The model under review builds one solid part; all positions refer to its coordinate system, in mm. Face numbers are marked on the shaded views. A direction names the side the tool comes from. Coordinates: 2 decimals unless noted, no trailing zeros. Write each loop counter-clockwise with the first axis right and the second up, starting at its lowest first coordinate (ties: lowest second). Pieces come first, ordered by that corner, then holes. Notation, with made-up numbers: (21, 86.25) - (50, 86.25) arc R20 cw to (50, 111.25) - close; hole circle Ø6 at (-13, 7). An arc over 180 degrees is marked (long way). Return JSON: item names as keys, results as strings. Group by question number.
(1) We need section A-A on z = -15. State the section outline as (x, y) points, then the cut area to 3 significant figures.
(2) We need section C-C on y = 3. State the section outline as (x, z) points, then the cut area to 3 significant figures.
(3) To check wall thickness, follow L1, parallel to X at y = 29, z = -6; L2, parallel to Y at x = 3, z = -28. State the ranges of each line that lie inside material, in increasing order. Write a range as from..to.
(4) We need section B-B on x = 10. State the section outline as (y, z) points, then the cut area to 3 significant figures.
(5) Tool access review of the marked faces 1 and 2: name each direction out of +Z, -Z, +X, -X, +Y, -Y from which nothing blocks a thin tool from reaching the whole face with its end or side.
(6) For pin 1 Ø10 at (y, z) = (23, -22.5) entering from +X; pin 2 Ø3 at (x, y) = (7, 35) entering from -Z, all flat-tipped, find the tip position at first contact; note any pin that passes through.
(7) We need section D-D on z = -7. State the section outline as (x, y) points, then the cut area to 3 significant figures.
```python
from build123d import *

# Parameters (mm, degrees)
F1_DEPTH = 30
F3_DEPTH = 15.3
F5_DEPTH = 25


with BuildPart() as f1:
    # F0 (on Top) → F1 (new body)
    with BuildSketch(Plane.XY):
        Polygon((4.9999998882, 40), (0, 40), (0, 0), (40, 0), (40, 4.9999998882), (4.9999998882, 4.9999998882), align=None)
    extrude(amount=-F1_DEPTH)

    # F2 (on face) → F3 (cut)
    with BuildSketch(Plane.YZ.offset(4.9999998882)):
        with BuildLine():
            Line((40, -3.8196602917), (40, 0))
            Line((40, 0), (29.9999997997, 0))
            ThreePointArc((29.9999997997, 0), (35.3523312718, -0.9874146635), (40, -3.8196602917))
        make_face()
        with BuildLine():
            Line((40, -30), (40, -26.1803397083))
            ThreePointArc((40, -26.1803397083), (35.3523313132, -29.0125853207), (29.9999998882, -30))
            Line((29.9999998882, -30), (40, -30))
        make_face()
    extrude(amount=-F3_DEPTH, mode=Mode.SUBTRACT)

    # F4 (on face) → F5 (cut)
    with BuildSketch(Plane(origin=(0, 4.9999998882, 0), x_dir=(-1, 0, 0), z_dir=(0, 1, 0))):
        with BuildLine():
            Line((-24.5546065271, 0), (-40, 0))
            Line((-40, 0), (-40, -30))
            Line((-40, -30), (-24.5546074611, -30))
            ThreePointArc((-24.5546074611, -30), (-39.5546074611, -14.999999533), (-24.5546065271, 0))
        make_face()
    extrude(amount=-F5_DEPTH, mode=Mode.SUBTRACT)


solid = f1.part
```
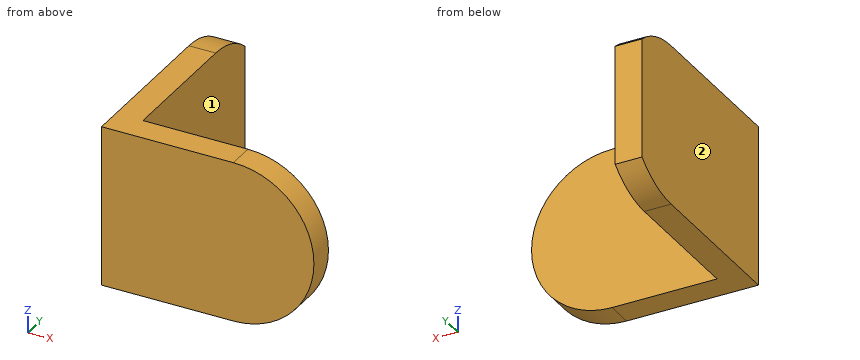
Ans:
{
 "1": {"outline": "(0, 0) - (39.55, 0) - (39.55, 5) - (5, 5) - (5, 40) - (0, 40) - close", "area": "373 mm²"},
 "2": {"outline": "(0, -30) - (24.55, -30) arc R15 ccw to (24.55, 0) - (0, 0) - close", "area": "1,090 mm²"},
 "3": {"L1": "0..5", "L2": "0..37.48"},
 "4": {"outline": "(0, -30) - (5, -30) - (5, 0) - (0, 0) - close", "area": "150 mm²"},
 "5": {"face 1": "+Z, -Z, +X, +Y", "face 2": "+Z, -Z, -X, +Y, -Y"},
 "6": {"pin 1": "x = 5", "pin 2": "through"},
 "7": {"outline": "(0, 0) - (37.24, 0) - (37.24, 5) - (5, 5) - (5, 40) - (0, 40) - close", "area": "361 mm²"}
}
